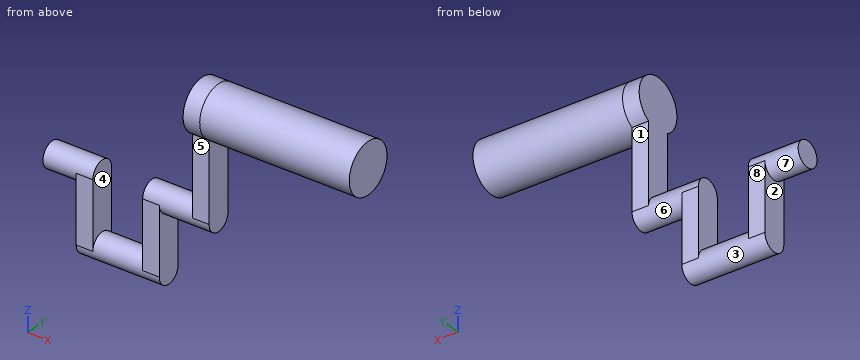
from build123d import *

# Parameters (mm, degrees)
SKETCH1_R           = 19.05
BOSS_EXTRUDE1_DEPTH = 127
BOSS_EXTRUDE2_START = -12.7
SKETCH2_R           = 9.525000000000007
BOSS_EXTRUDE2_DEPTH = 12.7
SKETCH2_3_R         = 9.525000000000007
BOSS_EXTRUDE3_DEPTH = 38.1
BOSS_EXTRUDE4_START = -12.7
SKETCH3_R           = 9.525000000000007
BOSS_EXTRUDE4_DEPTH = 12.7
SKETCH3_3_R         = 9.525000000000007
BOSS_EXTRUDE5_DEPTH = 50.8
BOSS_EXTRUDE6_START = 38.099999999999994
SKETCH3_4_R         = 9.525000000000007
BOSS_EXTRUDE6_DEPTH = 12.7
BOSS_EXTRUDE7_START = 88.9
SKETCH2_4_R         = 9.525000000000007
BOSS_EXTRUDE7_DEPTH = 25.4


with BuildPart() as part:
    # Sketch1 → Boss-Extrude1 (new body)
    with BuildSketch(Plane(origin=(0, 0, 0), x_dir=(0, 0, -1), z_dir=(1, 0, 0))):
        Circle(SKETCH1_R)
    extrude(amount=-BOSS_EXTRUDE1_DEPTH)

    # Sketch2 → Boss-Extrude2 (add)
    with BuildSketch(Plane.ZY.offset(127).offset(BOSS_EXTRUDE2_START)):
        with BuildLine():
            Line((-16.497783942092994, 9.525000000000002), (-76.2, 9.525000000000007))
            ThreePointArc((-76.2, 9.525000000000007), (-69.46480790919813, 6.73519209080187), (-66.675, 0))
            ThreePointArc((-66.675, -2.33e-15), (-69.46480790919813, -6.735192090801872), (-76.2, -9.525000000000007))
            Line((-76.2, -9.525000000000007), (-16.497783942092994, -9.525000000000002))
            ThreePointArc((-16.49778394209321, -9.525000000000603), (-19.05, 2.33e-15), (-16.497783942093204, 9.525000000000615))
        make_face()
        with BuildLine():
            ThreePointArc((19.05, 0), (4.930502809203364, 18.400886990806658), (-16.497783942093204, 9.525000000000615))
            Line((-16.497783942092994, 9.525000000000002), (0, 9.525))
            Line((0, 9.525), (0, -9.525))
            Line((0, -9.525), (-16.497783942092994, -9.525000000000002))
            ThreePointArc((-16.49778394209321, -9.525000000000603), (4.930502809203355, -18.40088699080666), (19.05, -4.67e-15))
        make_face()
        with BuildLine():
            Line((0, 9.525), (-16.497783942092994, 9.525000000000002))
            ThreePointArc((-16.497783942093204, 9.525000000000615), (-19.05, 2.33e-15), (-16.49778394209321, -9.525000000000603))
            Line((-16.497783942092994, -9.525000000000002), (0, -9.525))
            Line((0, -9.525), (0, 9.525))
        make_face()
        with Locations((-76.2, 0)):
            Circle(SKETCH2_R)
    extrude(amount=BOSS_EXTRUDE2_DEPTH)

    # Sketch2<3> → Boss-Extrude3 (add)
    with BuildSketch(Plane.ZY.offset(127)):
        with Locations((-76.2, 0)):
            Circle(SKETCH2_3_R)
    extrude(amount=BOSS_EXTRUDE3_DEPTH)

    # Sketch3 → Boss-Extrude4 (add)
    with BuildSketch(Plane.ZY.offset(165.1).offset(BOSS_EXTRUDE4_START)):
        with BuildLine():
            Line((-76.2, 9.525000000000007), (-127, 9.525000000000007))
            ThreePointArc((-127, 9.525000000000007), (-120.26480790919813, 6.73519209080187), (-117.475, 0))
            ThreePointArc((-117.475, -2.33e-15), (-120.26480790919813, -6.735192090801872), (-127, -9.525000000000007))
            Line((-127, -9.525000000000007), (-76.2, -9.525000000000007))
            ThreePointArc((-76.2, -9.525000000000006), (-85.72500000000001, 1.17e-15), (-76.2, 9.525000000000006))
        make_face()
        with Locations((-127, 0)):
            Circle(SKETCH3_R)
    extrude(amount=BOSS_EXTRUDE4_DEPTH)

    # Sketch3<3> → Boss-Extrude5 (add)
    with BuildSketch(Plane.ZY.offset(165.1)):
        with Locations((-127, 0)):
            Circle(SKETCH3_3_R)
    extrude(amount=BOSS_EXTRUDE5_DEPTH)

    # Sketch3<4> → Boss-Extrude6 (add)
    with BuildSketch(Plane.ZY.offset(165.1).offset(BOSS_EXTRUDE6_START)):
        with BuildLine():
            Line((-76.2, 9.525000000000007), (-127, 9.525000000000007))
            ThreePointArc((-127, 9.525000000000007), (-120.26480790919813, 6.73519209080187), (-117.475, 0))
            ThreePointArc((-117.475, -2.33e-15), (-120.26480790919813, -6.735192090801872), (-127, -9.525000000000007))
            Line((-127, -9.525000000000007), (-76.2, -9.525000000000007))
            ThreePointArc((-76.2, -9.525000000000006), (-85.72500000000001, 1.17e-15), (-76.2, 9.525000000000006))
        make_face()
        with Locations(Location((-76.2, 0, 0), (0, 0, 90))):
            Circle(SKETCH3_4_R)
    extrude(amount=BOSS_EXTRUDE6_DEPTH)

    # Sketch2<4> → Boss-Extrude7 (add)
    with BuildSketch(Plane.ZY.offset(127).offset(BOSS_EXTRUDE7_START)):
        with Locations(Location((-76.2, 0, 0), (0, 0, 90))):
            Circle(SKETCH2_4_R)
    extrude(amount=BOSS_EXTRUDE7_DEPTH)


solid = part.part
Verification items for the finished model (mm, model axes). Face numbers are marked on the shaded views. A direction names the side the tool comes from. Round coordinates to 2 decimals unless told otherwise and drop trailing zeros. Loops run counter-clockwise (first coordinate to the right, second up) from the corner with the lowest first, then second, coordinate; pieces in that order, holes last. Notation, with made-up numbers: (77, 5) - (134, 5) arc R13 ccw to (134, 23) - close; hole circle Ø9 at (37.5, 71.5). An arc over 180 degrees is marked (long way). Use a Markdown table: item, result. Add a question column.
1. Section check C-C, the plane x = -170. Record the boundary of the cut face in (y, z) (3 decimals), plus the area to 3 significant figures.
2. Section check D-D, the plane x = -86. Record the boundary of the cut face in (y, z), plus the area to 3 significant figures.
3. Thickness scan on probe 1 along X at (y, z) = (2, -73); probe 2 along X at (y, z) = (9, -84.5); probe 3 along Z at (x, y) = (-47.5, 16.5). Record the ranges inside material, lowest first. Write a range as [from, to].
4. Section check A-A, the plane y = 0. Record the boundary of the cut face in (x, z) (3 decimals), plus the area to 3 significant figures.
5. Gauge pin test, flat ends, axial feed: pin 1 (14 mm diameter, centred on x = -119.5, z = -38.5, fed in from -Y) (3 decimals); pin 2 (10 mm diameter, centred on x = -161, z = -97.5, fed in from +Y) (3 decimals); pin 3 (4 mm diameter, centred on y = 5.5, z = -24, fed in from +X). Record the tip position at first contact, or that the pin passes through.
6. Access from +Z, -Z, +X, -X, +Y, -Y to the whole of each face (thin tool, end or side, straight path). Record for the marked faces 5, 6, 7 and 8.
7. Section check B-B, the plane z = 0. Record the boundary of the cut face in (x, y), plus the area to 3 significant figures.
8. Release check for a two-part mould opening along X. For the marked faces 1, 2, 3 and 4 record: released by +X, released by -X, zero draft, split by the parting line, or undercut.
Checks:
| question | item | result |
|---|---|---|
| 1 | outline | circle Ø19.05 at (0, -127) |
| 1 | area | 285 mm^2 |
| 2 | outline | circle Ø38.1 at (0, 0) |
| 2 | area | 1,140 mm^2 |
| 3 | probe 1 | x = [-241.3, -203.2], [-165.1, -114.3] |
| 3 | probe 2 | x = [-215.9, -203.2], [-165.1, -152.4] |
| 3 | probe 3 | z = [-9.52, 9.52] |
| 4 | outline | (-241.3, -85.725) - (-215.9, -85.725) - (-215.9, -136.525) - (-152.4, -136.525) - (-152.4, -85.725) - (-114.3, -85.725) - (-114.3, -19.05) - (0, -19.05) - (0, 19.05) - (-127, 19.05) - (-127, -66.675) - (-165.1, -66.675) - (-165.1, -117.475) - (-203.2, -117.475) - (-203.2, -66.675) - (-241.3, -66.675) - close |
| 4 | area | 9,150 mm^2 |
| 5 | pin 1 | stops at y = -9.525 |
| 5 | pin 2 | stops at y = 9.525 |
| 5 | pin 3 | stops at x = -114.3 |
| 6 | face 5 | -Z, +X, -X, -Y |
| 6 | face 6 | none |
| 6 | face 7 | -X |
| 6 | face 8 | +Z, -Z, +X, -X, +Y |
| 7 | outline | (-127, -19.05) - (0, -19.05) - (0, 19.05) - (-127, 19.05) - close |
| 7 | area | 4,840 mm^2 |
| 8 | face 1 | zero draft |
| 8 | face 2 | released by -X |
| 8 | face 3 | undercut |
| 8 | face 4 | undercut |
